from build123d import *

# Parameters (mm, degrees)
F1_DEPTH = 40.64
F2_SIZE  = 25.4
F3_R     = 16.51
F4_DEPTH = 160.02
F5_R     = 13.97
F6_DEPTH = 33.02


with BuildPart() as f1:
    # F0 (on Front) → F1 (new body, symmetric)
    with BuildSketch(Plane.XZ):
        Polygon((-143.51, -43.18), (-31.75, -43.18), (-31.75, 0), (0, 0), (31.75, 0), (31.75, -43.18), (143.51, -43.18), (143.51, -10.16), (80.01, -10.16), (80.01, 139.7), (31.75, 139.7), (31.75, 33.02), (-31.75, 33.02), (-31.75, 139.7), (-80.01, 139.7), (-80.01, -10.16), (-143.51, -10.16), align=None)
    extrude(amount=F1_DEPTH, both=True)

    # F2
    f2_edges = [f1.edges().sort_by_distance(p)[0] for p in [
        (143.51, -40.64, -26.67),
        (-143.51, -40.64, -26.67),
    ]]
    chamfer(f2_edges, length=F2_SIZE)

    # F3 (on face) → F4 (cut)
    with BuildSketch(Plane.YZ.offset(80.01)):
        with BuildLine():
            ThreePointArc((-40.64, 119.38), (0, 129.212937), (40.64, 119.38))
            Line((40.64, 119.38), (40.64, 139.7))
            Line((40.64, 139.7), (-40.64, 139.7))
            Line((-40.64, 139.7), (-40.64, 119.38))
        make_face()
        with Locations((0, 73.66)):
            Circle(F3_R)
    extrude(amount=-F4_DEPTH, mode=Mode.SUBTRACT)

    # F5 (on face) → F6 (cut)
    with BuildSketch(Plane.XY.offset(-10.16)):
        with Locations((110.49, 7.62)):
            Circle(F5_R)
        with Locations((-110.49, 7.62)):
            Circle(F5_R)
    extrude(amount=-F6_DEPTH, mode=Mode.SUBTRACT)


solid = f1.part
Can you work these out from the model? Positions are in its coordinate system, mm. A direction names the side the tool comes from. Round coordinates to 2 decimals unless told otherwise and drop trailing zeros. Order: outer loops, then holes, each group sorted by start corner. A loop starts at its lowest first (then second) coordinate and runs counter-clockwise, first axis right, second up. Notation, with made-up numbers: (9.5, 32) - (45.5, 32) arc R17 cw to (45.5, 57) - close; hole circle Ø3 at (-31.5, -31.75). An arc over 180 degrees is marked (long way). Answer in a Markdown table with one row per item.
(1) Please list where these lines run through material, in increasing order: L1, parallel to Z at x = -65, y = 0; L2, parallel to X at y = 21, z = 113.5; L3, parallel to Y at x = 110.49, z = -21. Write a range as from..to.
From the geometry:
| item | result |
|---|---|
| L1 | z = -43.18..57.15, 90.17..129.21 |
| L2 | x = -80.01..-31.75, 31.75..80.01 |
| L3 | y = -40.64..-6.35, 21.59..40.64 |
(2) If we mould it in two halves opening along X, with no side actions, what happens to faces 6 (the face through (130.63, -28.12, -26.9)), 7 (the face through (-2, 40.64, 21)), 8 (the face through (0, -1, 0))? For each: released by +X, released by -X, zero draft, split by the parting line, or undercut.
From the geometry:
| item | result |
|---|---|
| face 6 | released by +X |
| face 7 | zero draft |
| face 8 | undercut |
(3) Suppose I cut it at D-D, the plane y = 0. Count the separate pieces of the cut face and the enclosed holes in it, plus the area to 3 significant figures.
From the geometry:
| item | result |
|---|---|
| separate pieces | 5 |
| enclosed holes | 0 |
| area | 18,200 mm2 |
(4) Which directions (+Z, -Z, +X, -X, +Y, -Y) give clear straight access to the entire face, cutting with the end or side of a thin tool? Please do faces 1 (the face through (31.75, -1, 92)), 2 (the face through (-55.54, 8.88, 87.58)), 3 (the face through (-80.01, -1, 45)), 4 (the face through (-31.75, -1, -22)), 5 (the face through (112, -10, -10.16)).
From the geometry:
| item | result |
|---|---|
| face 1 | +Z, +Y, -Y |
| face 2 | +X, -X |
| face 3 | +Z, -X, +Y, -Y |
| face 4 | -Z, +Y, -Y |
| face 5 | +Z, +X, +Y, -Y |
(5) Suppose I cut it at C-C, the plane z = 73.66. Please give me the cut outline in (x, y).
From the geometry:
| item | result |
|---|---|
| outline | (-80.01, -40.64) - (-31.75, -40.64) - (-31.75, -16.51) - (-80.01, -16.51) - close; (-80.01, 16.51) - (-31.75, 16.51) - (-31.75, 40.64) - (-80.01, 40.64) - close; (31.75, -40.64) - (80.01, -40.64) - (80.01, -16.51) - (31.75, -16.51) - close; (31.75, 16.51) - (80.01, 16.51) - (80.01, 40.64) - (31.75, 40.64) - close |
(6) Suppose I cut it at B-B, the plane z = 101. Please give me the cut outline in (x, y).
From the geometry:
| item | result |
|---|---|
| outline | (-80.01, -40.64) - (-31.75, -40.64) - (-31.75, 40.64) - (-80.01, 40.64) - close; (31.75, -40.64) - (80.01, -40.64) - (80.01, 40.64) - (31.75, 40.64) - close |
(7) For P1, Ø24.5, axis at y = -12, z = 80, coming from the -X side; P2, Ø5, axis at y = -11, z = 66, coming from the -X side; P3, Ø19, axis at x = -110.5, y = -4, coming from the +Z side; P4, Ø24.5, axis at y = 15, z = 62, coming from the +X side, each with a flat end and sliding along its axis, tell me the tip position at first contact or that it passes through.
From the geometry:
| item | result |
|---|---|
| P1 | stops at x = -80.01 |
| P2 | passes through |
| P3 | stops at z = -10.16 |
| P4 | stops at x = 80.01 |
(8) Suppose I cut it at A-A, the plane x = -110.49. Please give me the cut outline in (y, z).
From the geometry:
| item | result |
|---|---|
| outline | (-40.64, -43.18) - (-6.35, -43.18) - (-6.35, -10.16) - (-40.64, -10.16) - close; (21.59, -43.18) - (40.64, -43.18) - (40.64, -10.16) - (21.59, -10.16) - close |
